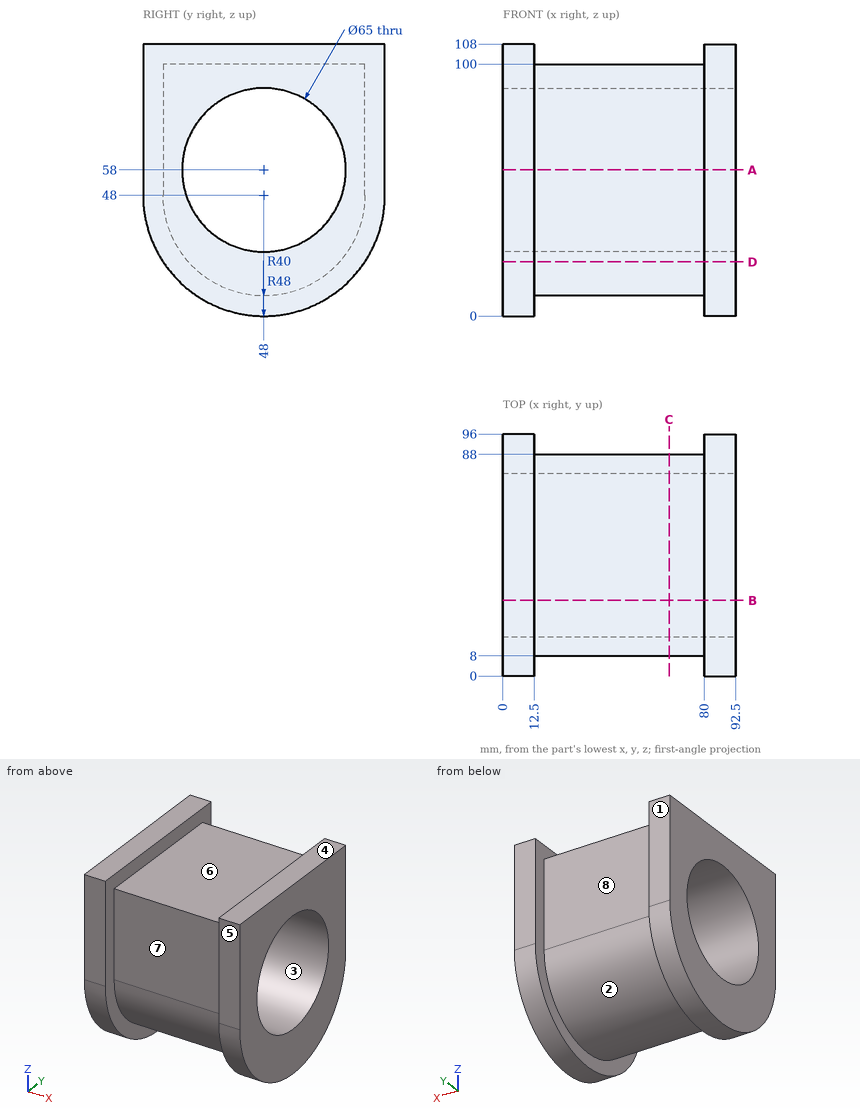
Verification items for this drawing (mm, ordinates from the low corner). A direction names the side the tool comes from. Coordinates: 2 decimals unless noted, no trailing zeros. Order: outer loops, then holes, each group sorted by start corner. A loop starts at its lowest first (then second) coordinate and runs counter-clockwise, first axis right, second up. Notation, with made-up numbers: (54, -12) -> (103, -12) arc R13 cw to (103, 8) -> close; hole circle Ø6 at (35, 2.5). An arc over 180 degrees is marked (long way). Answer as CSV lines item,"result". Start each with the question number.
1) Release check for a two-part mould opening along Z. For the marked faces 1, 2, 3 and 4 record: released by +Z, released by -Z, zero draft, split by the parting line, or undercut.
2) Gauge pin test, flat ends, axial feed: pin 1 Ø1 at (x, y) = (26, 78) entering from -Z; pin 2 Ø4 at (x, y) = (15.5, 32) entering from -Z; pin 3 Ø6 at (x, z) = (65, 61) entering from +Y. Record the tip position at first contact, or that the pin passes through.
3) Cross-section at B-B, the plane y = 30. Record the boundary of the cut face in (x, z), then the cut area to 3 significant figures.
4) Set-up check for the marked faces 5, 6, 7 and 8: record each of +Z, -Z, +X, -X, +Y, -Y from which the full face is reachable in a straight line by a thin tool's end or side.
5) Cross-section at C-C, the plane x = 66. Record the boundary of the cut face in (y, z), then the cut area to 3 significant figures.
6) Cross-section at A-A, the plane z = 58. Record the boundary of the cut face in (x, y), then the cut area to 3 significant figures.
7) Material ranges on L1, parallel to X at y = 29.5, z = 9; L2, parallel to Y at x = 41, z = 58; L3, parallel to Z at x = 19, y = 37, recorded low to high. Write a range as [from, to].
8) Cross-section at D-D, the plane z = 21.5. Record the boundary of the cut face in (x, y).
Conclusion:
1,face 1,"zero draft"
1,face 2,"released by -Z"
1,face 3,"undercut"
1,face 4,"released by +Z"
2,pin 1,"stops at z = 20.99"
2,pin 2,"stops at z = 10.53"
2,pin 3,"stops at y = 88"
3,outline,"(0, 3.5) -> (12.5, 3.5) -> (12.5, 12.28) -> (80, 12.28) -> (80, 3.5) -> (92.5, 3.5) -> (92.5, 30.94) -> (0, 30.94) -> close; (0, 85.06) -> (92.5, 85.06) -> (92.5, 108) -> (80, 108) -> (80, 100) -> (12.5, 100) -> (12.5, 108) -> (0, 108) -> close"
3,area,"3,530 mm²"
4,face 5,"+Z, -Z, +X, -X, -Y"
4,face 6,"+Z, +Y, -Y"
4,face 7,"+Z, -Z, -Y"
4,face 8,"+Z, -Z, +Y"
5,outline,"(8, 48) arc R40 ccw to (88, 48) -> (88, 100) -> (8, 100) -> close; hole circle Ø65 at (48, 58)"
5,area,"3,350 mm²"
6,outline,"(0, 0) -> (12.5, 0) -> (12.5, 8) -> (80, 8) -> (80, 0) -> (92.5, 0) -> (92.5, 15.5) -> (0, 15.5) -> close; (0, 80.5) -> (92.5, 80.5) -> (92.5, 96) -> (80, 96) -> (80, 88) -> (12.5, 88) -> (12.5, 96) -> (0, 96) -> close"
6,area,"1,790 mm²"
7,L1,"x = [0, 12.5], [80, 92.5]"
7,L2,"y = [8, 15.5], [80.5, 88]"
7,L3,"z = [9.54, 27.42], [88.58, 100]"
8,outline,"(0, 7.98) -> (12.5, 7.98) -> (12.5, 18.04) -> (80, 18.04) -> (80, 7.98) -> (92.5, 7.98) -> (92.5, 88.02) -> (80, 88.02) -> (80, 77.96) -> (12.5, 77.96) -> (12.5, 88.02) -> (0, 88.02) -> close"
